Check sheet for the modelled part. Datum: model origin and axes. Units: mm. Face numbers are marked on the shaded views. A direction names the side the tool comes from. Give positions to 0.01 mm unless a question says otherwise; leave off trailing zeros. Loops run counter-clockwise (first coordinate to the right, second up) from the corner with the lowest first, then second, coordinate; pieces in that order, holes last. Notation, with made-up numbers: (89.25, -4.5) -> (95.25, -4.5) arc R23 cw to (95.25, 13.5) -> close; hole circle Ø10 at (9, 5.5). An arc over 180 degrees is marked (long way). Answer as CSV lines item,"result". Start each with the question number.
(1) Release check for a two-part mould opening along Y. For the marked faces 1, 2 and 3 record: pulls with the +Y half, pulls with the -Y half, needs draft (parallel to the pull), parting line crosses it, or undercut.
(2) Access from +Z, -Z, +X, -X, +Y, -Y to the whole of each face (thin tool, end or side, straight path). Record for the marked faces 4, 5, 6 and 7.
(3) Section check C-C on y = 107. Enter the section's corners in (x, z), plus the area to 3 significant figures.
(4) Material ranges on line 1 (X direction, y = 18, z = 0); line 2 (Y direction, x = -10, z = 12); line 3 (X direction, y = 8, z = 0), recorded low to high. Write a range as from..to.
(5) Gauge pin test, flat ends, axial feed: pin 1 Ø17.5 at (x, y) = (3.5, 121) entering from +Z; pin 2 Ø2 at (y, z) = (118, 8) entering from +X; pin 3 Ø3 at (x, z) = (-24.5, 0.5) entering from +Y; pin 4 Ø5.5 at (x, z) = (-39, 0) entering from +Y. Record the tip position at first contact, or that the pin passes through.
(6) Section check B-B on y = 201.2. Enter the section's corners in (x, z), plus the area to 3 significant figures.
(7) Section check A-A on z = 0. Enter the section's corners in (x, y), plus the area to 3 significant figures.
from build123d import *

# Parameters (mm, degrees)
SKETCH1_R               = 28.232840849
SKETCH1_R_2             = 21.20600046
BOSS_EXTRUDE1_DEPTH     = 19
BOSS_EXTRUDE1_2_DEPTH   = 19
BOSS_EXTRUDE2_DEPTH     = 9
FILLET1_R               = 22.5
FILLET2_R               = 40
CUT_EXTRUDE_THIN1_DEPTH = 2
BOSS_EXTRUDE3_DEPTH     = 30
SKETCH5_R               = 4.5
CUT_EXTRUDE1_DEPTH      = 30
CUT_EXTRUDE2_DEPTH      = 30
FILLET3_R               = 3


with BuildPart() as part:
    # Sketch1 → Boss-Extrude1 (new, symmetric)
    with BuildSketch(Plane.XY):
        with Locations((0, 201.2)):
            Circle(SKETCH1_R)
        with Locations((0, 201.2)):
            Circle(SKETCH1_R_2, mode=Mode.SUBTRACT)
    extrude(amount=BOSS_EXTRUDE1_DEPTH, both=True)



with BuildPart() as body_2:
    # Sketch1 → Boss-Extrude1 2 (new, symmetric)
    with BuildSketch(Plane.XY):
        with BuildLine():
            Line((-36, 0), (-27, 0))
            ThreePointArc((-27, 0), (0, 27), (27, 0))
            Line((27, 0), (36, 0))
            ThreePointArc((36, 0), (0, 36), (-36, 0))
        make_face()
    extrude(amount=BOSS_EXTRUDE1_2_DEPTH, both=True)


with BuildPart() as part_1:
    add(part.part)

    add(body_2.part)  # Boss-Extrude2 merges body 2
    # Sketch2 → Boss-Extrude2 (add, symmetric)
    with BuildSketch(Plane.XY):
        with BuildLine():
            Line((-10, 174.797475454), (-17.512343456, 31.453423132))
            ThreePointArc((-17.512343456, 31.453423132), (0, 36), (17.512343456, 31.453423132))
            Line((17.512343456, 31.453423132), (10, 174.797475454))
            ThreePointArc((10, 174.797475454), (0, 172.967159151), (-10, 174.797475454))
        make_face()
    extrude(amount=BOSS_EXTRUDE2_DEPTH, both=True)

    # Fillet1
    fillet1_edges = [part_1.edges().sort_by_distance(p)[0] for p in [
        (10, 174.797475454, 0),
        (-10, 174.797475454, 0),
    ]]
    fillet(fillet1_edges, radius=FILLET1_R)

    # Fillet2
    fillet2_edges = [part_1.edges().sort_by_distance(p)[0] for p in [
        (-17.512343456, 31.453423132, 0),
        (17.512343456, 31.453423132, 0),
    ]]
    fillet(fillet2_edges, radius=FILLET2_R)

    # Sketch3 → Cut-Extrude-Thin1 (cut, symmetric)
    with BuildSketch(Plane.XY.offset(9)):
        with BuildLine():
            Line((-9, 62.771407141), (-9, 152.771407141))
            ThreePointArc((-9, 152.771407141), (0, 161.771407141), (9, 152.771407141))
            Line((9, 152.771407141), (9, 62.771407141))
            ThreePointArc((9, 62.771407141), (0, 53.771407141), (-9, 62.771407141))
        make_face()
        with BuildLine():
            Line((-8, 62.771407141), (-8, 152.771407141))
            ThreePointArc((-8, 152.771407141), (0, 160.771407141), (8, 152.771407141))
            Line((8, 152.771407141), (8, 62.771407141))
            ThreePointArc((8, 62.771407141), (0, 54.771407141), (-8, 62.771407141))
        make_face(mode=Mode.SUBTRACT)
    extrude(amount=CUT_EXTRUDE_THIN1_DEPTH, both=True, mode=Mode.SUBTRACT)

    # Sketch4 → Boss-Extrude3 (add)
    with BuildSketch(Plane(origin=(0, 0, 0), x_dir=(1, 0, 0), z_dir=(0, 1, 0))):
        with BuildLine():
            Line((-39, 9), (39, 9))
            ThreePointArc((39, 9), (48, 0), (39, -9))
            Line((39, -9), (-39, -9))
            ThreePointArc((-39, -9), (-48, 0), (-39, 9))
        make_face()
    extrude(amount=BOSS_EXTRUDE3_DEPTH)

    # Sketch5 → Cut-Extrude1 (cut)
    with BuildSketch(Plane(origin=(0, 30, 0), x_dir=(1, 0, 0), z_dir=(0, 1, 0))):
        with Locations(Location((-39, 0, 0), (0, 0, 270))):
            Circle(SKETCH5_R)
        with Locations(Location((39, 0, 0), (0, 0, 270))):
            Circle(SKETCH5_R)
    extrude(amount=-CUT_EXTRUDE1_DEPTH, mode=Mode.SUBTRACT)

    # Sketch7 → Cut-Extrude2 (cut)
    with BuildSketch(Plane.XY.offset(9)):
        with BuildLine():
            Line((-27, 0), (27, 0))
            ThreePointArc((27, 0), (0, 27), (-27, 0))
        make_face()
    extrude(amount=-CUT_EXTRUDE2_DEPTH, mode=Mode.SUBTRACT)

    # Fillet3
    # the kernel refuses this fillet: 3 mm, written as the material it adds along each edge
    with BuildSketch(Plane(origin=(0, 0, -9), x_dir=(1, 0, 0), z_dir=(0, -1, 0))) as fillet3_piece_1_section:
        with BuildLine():
            CenterArc((36 + FILLET3_R, -FILLET3_R), FILLET3_R, 90, 90)
            Line((36 + FILLET3_R, 0), (36, 0))
            Line((36, 0), (36, -FILLET3_R))
        make_face()
    fillet3_piece_1 = revolve(axis=Axis((0, 0, -9), (0, 0, 1)), revolution_arc=180, mode=Mode.PRIVATE)
    fillet3_piece_1 = split(fillet3_piece_1, bisect_by=Plane(origin=(34.368782616, 30, -9.69889031), z_dir=(0, -1, 0)), keep=Keep.TOP, mode=Mode.PRIVATE)
    add(fillet3_piece_1)
    with BuildSketch(Plane(origin=(0, 0, -9), x_dir=(1, 0, 0), z_dir=(0, -1, 0))) as fillet3_piece_2_section:
        with BuildLine():
            CenterArc((36 + FILLET3_R, -FILLET3_R), FILLET3_R, 90, 90)
            Line((36 + FILLET3_R, 0), (36, 0))
            Line((36, 0), (36, -FILLET3_R))
        make_face()
    fillet3_piece_2 = revolve(axis=Axis((0, 0, -9), (0, 0, 1)), revolution_arc=180, mode=Mode.PRIVATE)
    fillet3_piece_2 = fillet3_piece_2 - Plane(origin=(-56.554925494, 50.769482983, -9.84745497), x_dir=(0.9986295347545739, -0.05233595624294397, 0), z_dir=(0, 0, -1)) * Cylinder(40, 156, mode=Mode.PRIVATE)
    fillet3_piece_2 = fillet3_piece_2 - Plane(origin=(56.554925494, 50.769482983, -9.84745497), x_dir=(-0.9986295347545739, -0.05233595624294397, 0), z_dir=(0, 0, -1)) * Cylinder(40, 156, mode=Mode.PRIVATE)
    add(fillet3_piece_2)
    with BuildSketch(Plane(origin=(0, 0, 9), x_dir=(-1, 0, 0), z_dir=(0, -1, 0))) as fillet3_piece_3_section:
        with BuildLine():
            CenterArc((36 + FILLET3_R, -FILLET3_R), FILLET3_R, 90, 90)
            Line((36, -FILLET3_R), (36, 0))
            Line((36, 0), (36 + FILLET3_R, 0))
        make_face()
    fillet3_piece_3 = revolve(axis=Axis((0, 0, 9), (0, 0, -1)), revolution_arc=180, mode=Mode.PRIVATE)
    fillet3_piece_3 = split(fillet3_piece_3, bisect_by=Plane(origin=(-34.368785519, 30, 9.698889588), z_dir=(0, -1, 0)), keep=Keep.TOP, mode=Mode.PRIVATE)
    add(fillet3_piece_3)
    with BuildSketch(Plane(origin=(0, 0, 9), x_dir=(-1, 0, 0), z_dir=(0, -1, 0))) as fillet3_piece_4_section:
        with BuildLine():
            CenterArc((36 + FILLET3_R, -FILLET3_R), FILLET3_R, 90, 90)
            Line((36, -FILLET3_R), (36, 0))
            Line((36, 0), (36 + FILLET3_R, 0))
        make_face()
    fillet3_piece_4 = revolve(axis=Axis((0, 0, 9), (0, 0, -1)), revolution_arc=180, mode=Mode.PRIVATE)
    fillet3_piece_4 = fillet3_piece_4 - Plane(origin=(-56.554925494, 50.769482983, 10.5000003), x_dir=(0.9986295347545739, -0.05233595624294397, 0), z_dir=(0, 0, -1)) * Cylinder(40, 156, mode=Mode.PRIVATE)
    fillet3_piece_4 = fillet3_piece_4 - Plane(origin=(56.554925494, 50.769482983, 10.5000003), x_dir=(-0.9986295347545739, -0.05233595624294397, 0), z_dir=(0, 0, -1)) * Cylinder(40, 156, mode=Mode.PRIVATE)
    add(fillet3_piece_4)


solid = part_1.part
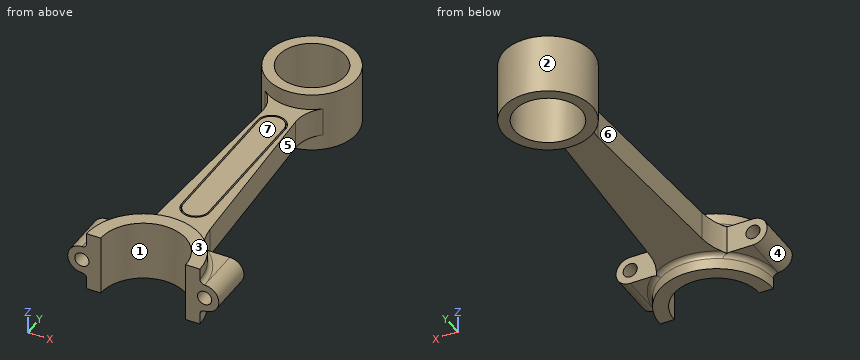
Working result:
1,face 1,"pulls with the -Y half"
1,face 2,"undercut"
1,face 3,"needs draft"
2,face 4,"-X, +Y, -Y"
2,face 5,"+Z, -Z, +X"
2,face 6,"+Z, -Z, -X"
2,face 7,"+Z, +X, -X"
3,outline,"(-13.55, -9) -> (13.55, -9) -> (13.55, 9) -> (9, 9) -> (9, 7) -> (8, 7) -> (8, 9) -> (-8, 9) -> (-8, 7) -> (-9, 7) -> (-9, 9) -> (-13.55, 9) -> close"
3,area,"484 mm^2"
4,line 1,"x = -48..-43.5, -34.5..-20.12, 20.12..34.5, 43.5..48"
4,line 2,"y = 25.08..34.58, 174.8..182.5, 219.9..227.6"
4,line 3,"x = -48..-43.5, -34.5..-25.79, 25.79..34.5, 43.5..48"
5,pin 1,"stops at z = 9"
5,pin 2,"stops at x = 13.03"
5,pin 3,"stops at y = 217.57"
5,pin 4,"passes through"
6,outline,"(-28.23, -19) -> (-21.21, -19) -> (-21.21, 19) -> (-28.23, 19) -> close; (21.21, -19) -> (28.23, -19) -> (28.23, 19) -> (21.21, 19) -> close"
6,area,"534 mm^2"
7,outline,"(-48, 0) -> (-43.5, 0) -> (-43.5, 30) -> (-48, 30) -> close; (-34.5, 0) -> (-27, 0) arc R27 cw to (27, 0) -> (34.5, 0) -> (34.5, 30) -> (22.37, 30) arc R40 cw to (16.61, 48.68) -> (10.69, 161.63) arc R22.5 cw to (18.45, 179.83) arc R28.23 ccw (long way) to (-18.45, 179.83) arc R22.5 cw to (-10.69, 161.63) -> (-16.61, 48.68) arc R40 cw to (-22.37, 30) -> (-34.5, 30) -> close; (43.5, 0) -> (48, 0) -> (48, 30) -> (43.5, 30) -> close; hole circle Ø42.41 at (0, 201.2)"
7,area,"6,360 mm^2"
